Design review of the part built by this model. Coordinates are the model's own, in mm. A direction names the side the tool comes from. Coordinates: 2 decimals unless noted, no trailing zeros. Write each loop counter-clockwise with the first axis right and the second up, starting at its lowest first coordinate (ties: lowest second). Pieces come first, ordered by that corner, then holes. Notation, with made-up numbers: (9, -32.5) - (32, -32.5) arc R25 ccw to (32, -1.5) - close; hole circle Ø4 at (-32, 8.25). An arc over 180 degrees is marked (long way). Answer as CSV lines item,"result". Start each with the question number.
Q1. For line 1 along Y through (x, z) = (255.5, 1); line 2 along Y through (x, z) = (256, 0.6); line 3 along X through (y, z) = (10.5, 2.6), list the stretches that pass through material, from the lowest coordinate up. Write a range as [from, to].
Q2. Machinability: for faces 4 (the face through (250.14, 85.76, 1.48)), 5 (the face through (318.314, 31.781, 1.479)), 6 (the face through (268, 46, 3)), which of the approach directions +Z, -Z, +X, -X, +Y, -Y give a long, thin tool a straight path to every point of the face, cutting with its end or side? Answer none if there is none.
Q3. We need section C-C (z = 1.35). State how many separate pieces and enclosed holes the cut face has, plus the area to 3 significant figures.
Q4. We need section B-B (y = 26.5). Write out the cut boundary in (x, z).
Q5. Mouldability with a two-part tool opening along X and no side actions: class faces 1 (the face through (268, 46, 0)), 2 (the face through (202.22, 53.88, 1.48)), 3 (the face through (259.25, 15.36, 1.48)) as pulls with the +X half, pulls with the -X half, needs draft (parallel to the pull), parting line crosses it, or undercut.
Q6. We need section D-D (x = 188). Write out the cut boundary in (y, z).
Q7. Clearance check with flat-ended pins moving along their axes: pin 1 (1.2 mm diameter, centred on x = 363.5, z = 1, fed in from -Y); pin 2 (5 mm diameter, centred on x = 246.5, y = 32, fed in from -Z) (1 decimal); pin 3 (4 mm diameter, centred on x = 295.5, y = 48, fed in from -Z); pin 4 (0.8 mm diameter, centred on x = 363, z = 2, fed in from +Y). State where each tip first meets the part, or that it passes through.
Q8. We need section A-A (x = 215.5). Write out the cut boundary in (y, z).
from build123d import *

# Parameters (mm, degrees)
SKETCH_1_R      = 2
SKETCH_1_R_2    = 5.5
EXTRUDE_1_DEPTH = 3


with BuildPart() as part:
    # 草图1 → 凸台-拉伸1 (new body)
    with BuildSketch(Plane.XY):
        with BuildLine():
            Line((234.002581869, 13.707860978), (182.002581869, 13.707860978))
            ThreePointArc((182.002581869, 13.707860978), (168.34572762, 8.051006728), (174.002581869, 21.707860978))
            Line((174.002581869, 21.707860978), (231.242343182, 86.967009497))
            ThreePointArc((231.242343182, 86.967009497), (238.565892024, 94.911259453), (249.002581869, 97.707860978))
            Line((249.002581869, 97.707860978), (354.002581869, 97.707860978))
            Line((354.002581869, 97.707860978), (364.002581869, 97.707860978))
            Line((364.002581869, 97.707860978), (364.002581869, 89.707860978))
            Line((364.002581869, 89.707860978), (361.502581869, 89.707860978))
            Line((361.502581869, 89.707860978), (361.502581869, 91.207860978))
            Line((361.502581869, 91.207860978), (358.902581869, 91.207860978))
            Line((358.902581869, 91.207860978), (358.902581869, 89.707860978))
            Line((358.902581869, 89.707860978), (355.902581869, 89.707860978))
            Line((355.902581869, 89.707860978), (355.902581869, 86.707860978))
            Line((355.902581869, 86.707860978), (358.902581869, 86.707860978))
            Line((358.902581869, 86.707860978), (358.902581869, 85.207860978))
            Line((358.902581869, 85.207860978), (361.502581869, 85.207860978))
            Line((361.502581869, 85.207860978), (361.502581869, 86.707860978))
            Line((361.502581869, 86.707860978), (364.002581869, 86.707860978))
            Line((364.002581869, 86.707860978), (364.002581869, 57.707860978))
            Line((364.002581869, 57.707860978), (367.002581869, 57.707860978))
            Line((367.002581869, 57.707860978), (367.002581869, 49.707860978))
            Line((367.002581869, 49.707860978), (364.002581869, 49.707860978))
            Line((364.002581869, 49.707860978), (364.002581869, 20.707860978))
            Line((364.002581869, 20.707860978), (361.502581869, 20.707860978))
            Line((361.502581869, 20.707860978), (361.502581869, 22.207860978))
            Line((361.502581869, 22.207860978), (358.902581869, 22.207860978))
            Line((358.902581869, 22.207860978), (358.902581869, 20.707860978))
            Line((358.902581869, 20.707860978), (355.902581869, 20.707860978))
            Line((355.902581869, 20.707860978), (355.902581869, 17.707860978))
            Line((355.902581869, 17.707860978), (358.902581869, 17.707860978))
            Line((358.902581869, 17.707860978), (358.902581869, 16.207860978))
            Line((358.902581869, 16.207860978), (361.502581869, 16.207860978))
            Line((361.502581869, 16.207860978), (361.502581869, 17.707860978))
            Line((361.502581869, 17.707860978), (364.002581869, 17.707860978))
            Line((364.002581869, 17.707860978), (364.002581869, 9.707860978))
            Line((364.002581869, 9.707860978), (355.16842929, 9.707860978))
            ThreePointArc((355.16842929, 9.707860978), (354.089046944, 9.908765811), (353.154233351, 10.484571811))
            ThreePointArc((353.154233351, 10.484571811), (317.768023154, 31.985283132), (276.929619495, 38.818236083))
            ThreePointArc((276.929619495, 38.818236083), (274.855620398, 37.914488932), (274.002581869, 35.819123465))
            Line((274.002581869, 35.819123465), (274.002581869, 13.707860978))
            ThreePointArc((274.002581869, 13.707860978), (254.002581869, -6.292139022), (234.002581869, 13.707860978))
        make_face()
        with Locations((174.002581869, 13.707860978)):
            Circle(SKETCH_1_R, mode=Mode.SUBTRACT)
        with Locations((254.002581869, 13.707860978)):
            Circle(SKETCH_1_R_2, mode=Mode.SUBTRACT)
        with BuildLine():
            Line((253.002581869, 86.967009497), (344.129272471, 86.967009497))
            ThreePointArc((344.129272471, 86.967009497), (346.957699596, 85.795436622), (348.129272471, 82.967009497))
            Line((348.129272471, 82.967009497), (348.129272471, 36.172406577))
            ThreePointArc((348.129272471, 36.172406577), (346.444858552, 32.910802508), (342.810241921, 32.396144085))
            Line((342.810241921, 32.396144085), (251.683551319, 64.226264226))
            ThreePointArc((251.683551319, 64.226264226), (249.740977801, 65.686940637), (249.002581869, 68.002526718))
            Line((249.002581869, 68.002526718), (249.002581869, 82.967009497))
            ThreePointArc((249.002581869, 82.967009497), (250.174154745, 85.795436622), (253.002581869, 86.967009497))
        make_face(mode=Mode.SUBTRACT)
        with BuildLine():
            Line((255.549578652, 43.172566622), (249.002581869, 45.970414811))
            Line((249.002581869, 45.970414811), (231.242343182, 53.560223281))
            ThreePointArc((231.242343182, 53.560223281), (229.530107584, 53.753780798), (227.993824006, 52.973365511))
            Line((227.993824006, 52.973365511), (208.259363433, 34.167429409))
            ThreePointArc((208.259363433, 34.167429409), (207.543711742, 30.881045102), (210.328975867, 28.99563191))
            Line((210.328975867, 28.99563191), (254.37067191, 28.99563191))
            ThreePointArc((254.37067191, 28.99563191), (256.491992253, 29.874311567), (257.37067191, 31.99563191))
            Line((257.37067191, 31.99563191), (257.37067191, 40.413911353))
            ThreePointArc((257.37067191, 40.413911353), (256.87434124, 42.066678695), (255.549578652, 43.172566622))
        make_face(mode=Mode.SUBTRACT)
    extrude(amount=EXTRUDE_1_DEPTH)


solid = part.part
Results list:
1,line 1,"y = [-6.24, 8.42], [19, 29.22], [43.19, 62.89], [86.97, 97.71]"
1,line 2,"y = [-6.19, 8.58], [18.83, 29.48], [42.93, 62.72], [86.97, 97.71]"
1,line 3,"x = [166.67, 181.33], [234.26, 249.53], [258.47, 273.74], [353.14, 364]"
2,face 4,"+Z, -Z"
2,face 5,"+Z, -Z, -Y"
2,face 6,"+Z, +X, -X, +Y, -Y"
3,separate pieces,"1"
3,enclosed holes,"4"
3,area,"8,040 mm2"
4,outline,"(178.21, 0) - (274, 0) - (274, 3) - (178.21, 3) - close; (330.13, 0) - (364, 0) - (364, 3) - (330.13, 3) - close"
5,face 1,"needs draft"
5,face 2,"pulls with the -X half"
5,face 3,"undercut"
6,outline,"(13.71, 0) - (37.67, 0) - (37.67, 3) - (13.71, 3) - close"
7,pin 1,"stops at y = 9.71"
7,pin 2,"passes through"
7,pin 3,"stops at z = 0"
7,pin 4,"stops at y = 97.71"
8,outline,"(13.71, 0) - (29, 0) - (29, 3) - (13.71, 3) - close; (41.07, 0) - (69.02, 0) - (69.02, 3) - (41.07, 3) - close"
